Model file for the job. Use its own axes, mm. Coordinates: 2 decimals unless noted, no trailing zeros. Write each loop counter-clockwise with the first axis right and the second up, starting at its lowest first coordinate (ties: lowest second). Pieces come first, ordered by that corner, then holes. Notation, with made-up numbers: (36.5, 43) - (45.5, 43) arc R20 ccw to (45.5, 74) - close; hole circle Ø5 at (68, 43.5). An arc over 180 degrees is marked (long way). Put each result on its own line as item: value. Start each with the question number.
1. Saw through at C-C, the plane z = 1. Write the cut outline in (x, y).
2. Drill centre lines: L1, parallel to Y at x = 8, z = -35; L2, parallel to X at y = 1.75, z = 25; L3, parallel to Z at x = 10.75, y = -0.5. Where is each one in solid material? Low to high. Write a range as from..to.
3. Pull direction Y, two halves, no side cores. Call faces 1 (the face through (1.01, 0.04, 35.85)), 2 (the face through (7.4, -0.54, -37.44)), 3 (the face through (0, 0, -1)): released by +Y, released by -Y, zero draft, split by the parting line, or undercut.
4. Saw through at B-B, the plane x = 11. Write the cut outline in (y, z), plus the area to 3 significant figures.
5. Saw through at A-A, the plane y = 0. Write the cut outline in (x, z).
6. Drop flat-ended pins along their axis: P1, Ø1, axis at x = 10, y = -1, coming from the -Z side; P2, Ø2, axis at y = -2, z = 30, coming from the +X side; P3, Ø1.5, axis at x = 12, y = 1, coming from the -Z side. Give the stop position or say it passes through.
```python
from build123d import *

# Parameters (mm, degrees)
RESSALTO_EXTRUS_O1_DEPTH = 2
ESBO_O2_R                = 2.5
RESSALTO_EXTRUS_O2_DEPTH = 13
CORTE_EXTRUS_O1_REACH    = 42.466
ESBO_O3_R                = 0.85
CORTE_EXTRUS_O2_REACH    = 41.768
ESBO_O4_R                = 0.85


with BuildPart() as part:
    # Esboço1 → Ressalto-extrusão1 (new body)
    with BuildSketch(Plane(origin=(0, 0, 0), x_dir=(0, 0, -1), z_dir=(1, 0, 0))):
        with BuildLine():
            Line((-35, 2.5), (35, 2.5))
            ThreePointArc((35, 2.5), (37.5, 0), (35, -2.5))
            Line((35, -2.5), (-35, -2.5))
            ThreePointArc((-35, -2.5), (-37.5, 0), (-35, 2.5))
        make_face()
    extrude(amount=RESSALTO_EXTRUS_O1_DEPTH)

    # Esboço2 → Ressalto-extrusão2 (add)
    with BuildSketch(Plane(origin=(2, 0, 0), x_dir=(0, 0, -1), z_dir=(1, 0, 0))):
        with Locations(Location((35, 0, 0), (0, 0, 90))):
            Circle(ESBO_O2_R)
    extrude(amount=RESSALTO_EXTRUS_O2_DEPTH)

    # Esboço3 → Corte-extrusão1 (cut, up to next)
    with BuildSketch(Plane(origin=(15, 0, 0), x_dir=(0, 0, -1), z_dir=(1, 0, 0)), mode=Mode.PRIVATE) as corte_extrus_o1_sk1:
        with Locations((35, 0)):
            Circle(ESBO_O3_R)
    corte_extrus_o1_tool1 = extrude(corte_extrus_o1_sk1.sketch, amount=-CORTE_EXTRUS_O1_REACH, mode=Mode.PRIVATE) & part.part
    add(corte_extrus_o1_tool1.solids().sort_by_distance((15, 0, -35))[0], mode=Mode.SUBTRACT)

    # Esboço4 → Corte-extrusão2 (cut, up to next)
    with BuildSketch(Plane(origin=(2, 0, 0), x_dir=(0, 0, -1), z_dir=(1, 0, 0)), mode=Mode.PRIVATE) as corte_extrus_o2_sk1:
        with Locations((-35, 0)):
            Circle(ESBO_O4_R)
    corte_extrus_o2_tool1 = extrude(corte_extrus_o2_sk1.sketch, amount=-CORTE_EXTRUS_O2_REACH, mode=Mode.PRIVATE) & part.part
    add(corte_extrus_o2_tool1.solids().sort_by_distance((2, 0, 35))[0], mode=Mode.SUBTRACT)


solid = part.part
```
Final values:
1. outline: (0, -2.5) - (2, -2.5) - (2, 2.5) - (0, 2.5) - close
2. L1: y = -2.5..-0.85, 0.85..2.5
2. L2: x = 0..2
2. L3: z = -37.45..-35.69, -34.31..-32.55
3. face 1: undercut
3. face 2: split by the parting line
3. face 3: zero draft
4. outline: circle Ø5 at (0, -35); hole circle Ø1.7 at (0, -35)
4. area: 17.4 mm²
5. outline: (0, -37.5) - (15, -37.5) - (15, -35.85) - (0, -35.85) - close; (0, -34.15) - (15, -34.15) - (15, -32.5) - (2, -32.5) - (2, 34.15) - (0, 34.15) - close; (0, 35.85) - (2, 35.85) - (2, 37.5) - (0, 37.5) - close
6. P1: stops at z = -37.45
6. P2: stops at x = 2
6. P3: stops at z = -37.49
